Source: CAD feature listing. Evaluate the final solid. Frame: model axes, mm. A direction names the side the tool comes from. Round coordinates to 2 decimals unless told otherwise and drop trailing zeros. Order: outer loops, then holes, each group sorted by start corner. A loop starts at its lowest first (then second) coordinate and runs counter-clockwise, first axis right, second up. Notation, with made-up numbers: (52.5, -1) - (65.5, -1) arc R21 ccw to (65.5, 37) - close; hole circle Ø11 at (78.25, -1). An arc over 180 degrees is marked (long way). Put each result on its own line as item: value. Start each with the question number.
1) Access query for faces 4 (the face through (-91, 10, 7)), 5 (the face through (-100, 5, -2.95)), 6 (the face through (-19.27, 111.66, -4.77)), 7 (the face through (-6, 113, -5)), 8 (the face through (-79.817, 26.321, -17.469)). Directions: +Z, -Z, +X, -X, +Y, -Y. A direction counts if a zero-diameter tool reaches every point of the face in a straight line with its end or side. Return the directions, or none.
2) Contact query for flat-ended pins moving along their axis: P1, Ø1.5, axis at x = -100.5, z = 8, coming from the -Y side; P2, Ø8, axis at y = 94.5, z = -17, coming from the +X side; P3, Ø5, axis at y = 87.25, z = -5, coming from the -X side; P4, Ø10, axis at y = 35.5, z = 1.5, coming from the -X side. Output: stop coordinate, or through.
3) Line query: probe 1 along Y at (x, z) = (-4, 5); probe 2 along X at (y, z) = (9, 4.5); probe 3 along X at (y, z) = (62, 0). Output: solid intervals per line, ascending. Write a range as [from, to].
4) Section B-B on y = 98.5. Output: boundary loops of the cut face in (x, z), then the cut area to 3 significant figures.
5) Section D-D on x = -8.5. Output: boundary loops of the cut face in (y, z).
6) Section C-C on z = -33. Output: boundary loops of the cut face in (x, y), then the cut area to 3 significant figures.
7) Section A-A on z = -8.5. Output: boundary loops of the cut face in (x, y).
8) Mould query, pull axis Z, two halves, no side actions, for faces 1 (the face through (-20.288, 115.135, -4.709)), 2 (the face through (-91, 10, -6)), 3 (the face through (-100, 5, 2.95)). Classes: +Z half, -Z half, draft (parallel to the pull), parting line (faces both ways), or undercut.
```python
from build123d import *

# Parameters (mm, degrees)
BOSS_EXTRUDE1_DEPTH        = 10
SKETCH2_W                  = 5.05
SKETCH2_H                  = 7.05
CUT_EXTRUDE6_DEPTH         = 10
CUT_EXTRUDE7_DEPTH         = 5
CHAMFER2_SIZE              = 5.196152423
CHAMFER2_SIZE_2            = 9
CHAMFER2_OF_MIRROR4_SIZE   = 5.196152423
CHAMFER2_OF_MIRROR4_SIZE_2 = 9
SKETCH5_R                  = 2
CUT_EXTRUDE5_DEPTH         = 6
CUT_EXTRUDE8_START         = -120
CUT_EXTRUDE8_DEPTH         = 24.374622763
SKETCH8_R                  = 144.95
CUT_EXTRUDE9_DEPTH         = 12
BOSS_EXTRUDE2_DEPTH        = 20
SKETCH12_R                 = 2
CUT_EXTRUDE10_DEPTH        = 6
BOSS_EXTRUDE3_START        = -21
SKETCH13_W                 = 31.497171345
SKETCH13_H                 = 26
BOSS_EXTRUDE3_DEPTH        = 4
CHAMFER3_SIZE              = 15


# Read off the part's stored shape, not the designer's step: Cut-Extrude8
with BuildPart() as part:
    # Sketch1 → Boss-Extrude1 (new, symmetric)
    with BuildSketch(Plane.XY):
        Polygon((0, 120), (0, 80), (-10, 80), (-87.75, 12), (-87.75, 0), (-102.75, 0), (-102.75, 24), (-20, 120), align=None)
    extrude(amount=BOSS_EXTRUDE1_DEPTH, both=True)

    # Sketch2 → Cut-Extrude6 (cut)
    with BuildSketch(Plane.XZ):
        with Locations((-100.225, 6.475)):
            Rectangle(SKETCH2_W, SKETCH2_H)
        with Locations((-90.275, 6.475)):
            Rectangle(SKETCH2_W, SKETCH2_H)
        with Locations((-90.275, -6.475)):
            Rectangle(SKETCH2_W, SKETCH2_H)
        with Locations((-100.225, -6.475)):
            Rectangle(SKETCH2_W, SKETCH2_H)
    extrude(amount=-CUT_EXTRUDE6_DEPTH, mode=Mode.SUBTRACT)

    # Sketch6 → Cut-Extrude7 (cut)
    with BuildSketch(Plane.XY.offset(10)):
        Polygon((-98.494242528, 28.937192959), (-85.75, 13.749196141), (-13, 77.376205788), (-25.986145629, 113.055347669), align=None)
    cut_extrude7 = extrude(amount=-CUT_EXTRUDE7_DEPTH, mode=Mode.SUBTRACT)

    # Chamfer2
    # the kernel refuses this chamfer: 9, 5.196152423 mm, written as the material it adds along each edge
    with BuildSketch(Plane(origin=(-5.036481035, 55.496617251, 5), x_dir=(0.05440243528858507, 0.019800867116638043, 0.9983227437537925), z_dir=(-0.342020143325666, 0.9396926207859094, 0))) as chamfer2_piece_1_section:
        Polygon((CHAMFER2_SIZE * 0.998322743697, -CHAMFER2_SIZE * 0.0578938623994), (-CHAMFER2_SIZE_2 * 0.0578938624027, -CHAMFER2_SIZE_2 * 0.998322743754), (0, 0), align=None)
    chamfer2_piece_1 = extrude(amount=84.536493315, mode=Mode.PRIVATE)
    chamfer2_piece_1 = split(chamfer2_piece_1, bisect_by=Plane(origin=(-21.83844233, 92.842389445, 10), z_dir=(0, 0, -1)), keep=Keep.TOP, mode=Mode.PRIVATE)
    chamfer2_piece_1 = split(chamfer2_piece_1, bisect_by=Plane(origin=(-34.214088998, 103.509939047, 6.650101228), z_dir=(0.7574435982041207, -0.6529006015769894, 0)), keep=Keep.TOP, mode=Mode.PRIVATE)
    chamfer2_piece_1 = split(chamfer2_piece_1, bisect_by=Plane(origin=(-10.343648825, 79.699445401, 6.650101228), z_dir=(-0.6583332390976693, 0.7527266079388791, 0)), keep=Keep.TOP, mode=Mode.PRIVATE)
    add(chamfer2_piece_1)
    with BuildSketch(Plane(origin=(-113.460762542, 46.773596955, 5), x_dir=(-0.04434927158426045, -0.03721345742933334, 0.9983227437537927), z_dir=(0.642787609686533, -0.7660444431189835, 0))) as chamfer2_piece_2_section:
        Polygon((CHAMFER2_SIZE * 0.998322743697, -CHAMFER2_SIZE * 0.0578938623994), (-CHAMFER2_SIZE_2 * 0.0578938624027, -CHAMFER2_SIZE_2 * 0.998322743754), (0, 0), align=None)
    chamfer2_piece_2 = extrude(amount=66.394065339, mode=Mode.PRIVATE)
    chamfer2_piece_2 = split(chamfer2_piece_2, bisect_by=Plane(origin=(-97.520772346, 30.066536009, 6.631431033), z_dir=(0.7574435982041207, -0.6529006015769894, 0)), keep=Keep.TOP, mode=Mode.PRIVATE)
    chamfer2_piece_2 = split(chamfer2_piece_2, bisect_by=Plane(origin=(-83.277010041, 15.912068389, 6.631431033), z_dir=(-0.6583332390976693, 0.7527266079388791, 0)), keep=Keep.TOP, mode=Mode.PRIVATE)
    chamfer2_piece_2 = split(chamfer2_piece_2, bisect_by=Plane(origin=(-89.945880011, 23.537136627, 10), z_dir=(0, 0, -1)), keep=Keep.TOP, mode=Mode.PRIVATE)
    add(chamfer2_piece_2)

    # Mirror4: Cut-Extrude7 across plane
    add(cut_extrude7.mirror(Plane.XY), mode=Mode.SUBTRACT)

    # Chamfer2 of Mirror4
    # the kernel refuses this chamfer: 9, 5.196152423 mm, written as the material it adds along each edge
    with BuildSketch(Plane(origin=(-5.036481035, 55.496617251, -5), x_dir=(0.05440243528858507, 0.019800867116638043, -0.9983227437537925), z_dir=(-0.342020143325666, 0.9396926207859094, 0))) as chamfer2_of_mirror4_piece_1_section:
        Polygon((CHAMFER2_OF_MIRROR4_SIZE * 0.998322743697, CHAMFER2_OF_MIRROR4_SIZE * 0.0578938623994), (-CHAMFER2_OF_MIRROR4_SIZE_2 * 0.0578938624027, CHAMFER2_OF_MIRROR4_SIZE_2 * 0.998322743754), (0, 0), align=None)
    chamfer2_of_mirror4_piece_1 = extrude(amount=84.536493315, mode=Mode.PRIVATE)
    chamfer2_of_mirror4_piece_1 = split(chamfer2_of_mirror4_piece_1, bisect_by=Plane(origin=(-34.214088998, 103.509939047, -6.650101228), z_dir=(0.7574435982040639, -0.6529006015770552, 0)), keep=Keep.TOP, mode=Mode.PRIVATE)
    chamfer2_of_mirror4_piece_1 = split(chamfer2_of_mirror4_piece_1, bisect_by=Plane(origin=(-10.343648825, 79.699445401, -6.650101228), z_dir=(-0.6583332390977968, 0.7527266079387677, 0)), keep=Keep.TOP, mode=Mode.PRIVATE)
    chamfer2_of_mirror4_piece_1 = split(chamfer2_of_mirror4_piece_1, bisect_by=Plane(origin=(-21.83844233, 92.842389445, -10), z_dir=(0, 0, 1)), keep=Keep.TOP, mode=Mode.PRIVATE)
    add(chamfer2_of_mirror4_piece_1)
    with BuildSketch(Plane(origin=(-113.460762542, 46.773596955, -5), x_dir=(0.7659013618145366, 0.6426675502167433, 0.019326765612700778), z_dir=(0.642787609686533, -0.7660444431189835, 0))) as chamfer2_of_mirror4_piece_2_section:
        Polygon((CHAMFER2_OF_MIRROR4_SIZE_2 * 0.999813220622, -CHAMFER2_OF_MIRROR4_SIZE_2 * 0.0193267656127), (-CHAMFER2_OF_MIRROR4_SIZE * 0.0193267656116, -CHAMFER2_OF_MIRROR4_SIZE * 0.999813220566), (0, 0), align=None)
    chamfer2_of_mirror4_piece_2 = extrude(amount=66.394065339, mode=Mode.PRIVATE)
    chamfer2_of_mirror4_piece_2 = split(chamfer2_of_mirror4_piece_2, bisect_by=Plane(origin=(-97.520772346, 30.066536009, -6.631431033), z_dir=(0.7574435982040639, -0.6529006015770552, 0)), keep=Keep.TOP, mode=Mode.PRIVATE)
    chamfer2_of_mirror4_piece_2 = split(chamfer2_of_mirror4_piece_2, bisect_by=Plane(origin=(-83.277010041, 15.912068389, -6.631431033), z_dir=(-0.6583332390977968, 0.7527266079387677, 0)), keep=Keep.TOP, mode=Mode.PRIVATE)
    chamfer2_of_mirror4_piece_2 = split(chamfer2_of_mirror4_piece_2, bisect_by=Plane(origin=(-89.945880011, 23.537136627, -10), z_dir=(0, 0, 1)), keep=Keep.TOP, mode=Mode.PRIVATE)
    add(chamfer2_of_mirror4_piece_2)

    # Sketch5 → Cut-Extrude5 (cut)
    with BuildSketch(Plane(origin=(0, 0, 0), x_dir=(0, 0, -1), z_dir=(1, 0, 0))):
        with Locations((-5, 112.75)):
            Circle(SKETCH5_R)
        with Locations((-5, 87.25)):
            Circle(SKETCH5_R)
        with Locations(Location((5, 87.25, 0), (0, 0, 180))):
            Circle(SKETCH5_R)
        with Locations(Location((5, 112.75, 0), (0, 0, 180))):
            Circle(SKETCH5_R)
    extrude(amount=-CUT_EXTRUDE5_DEPTH, mode=Mode.SUBTRACT)

    # Cut-Extrude8 outline → Cut-Extrude8 (cut)
    with BuildSketch(Plane(origin=(0, 120, 0), x_dir=(1, 0, 0), z_dir=(0, 1, 0)).offset(CUT_EXTRUDE8_START)):
        with BuildLine():
            Line((-102.75, 7.56e-07), (-102.75, -10))
            Line((-102.75, -10), (-102.427082983, -10))
            ThreePointArc((-102.427082983, -10), (-102.669249724, -5.002605828), (-102.75, 7.56e-07))
        make_face()
        with BuildLine():
            Line((-102.427082983, 10), (-102.75, 10))
            Line((-102.75, 10), (-102.75, 7.56e-07))
            ThreePointArc((-102.75, 7.56e-07), (-102.669249699, 5.002606583), (-102.427082983, 10))
        make_face()
    extrude(amount=CUT_EXTRUDE8_DEPTH, mode=Mode.SUBTRACT)

    # Sketch8 → Cut-Extrude9 (cut)
    with BuildSketch(Plane.XZ):
        with Locations((56.25, 0)):
            Circle(SKETCH8_R)
    extrude(amount=-CUT_EXTRUDE9_DEPTH, mode=Mode.SUBTRACT)

    # Sketch10 → Boss-Extrude2 (add)
    with BuildSketch(Plane(origin=(0, 0, -10), x_dir=(-1, 0, 0), z_dir=(0, 0, -1))):
        Polygon((87.75, 12), (88.771540348, 10.230640215), (90.560927794, 10.230640215), (90.560927794, 12), align=None)
    extrude(amount=-BOSS_EXTRUDE2_DEPTH)

    # Sketch12 → Cut-Extrude10 (cut)
    with BuildSketch(Plane(origin=(-70.818661801, 61.044211083, 0), x_dir=(0, 0, 1), z_dir=(-0.7574435982041208, 0.6529006015769894, 0))):
        with Locations(Location((-4.797171345, 71.964164649, 0), (0, 0, 270))):
            Circle(SKETCH12_R)
        with Locations(Location((4.797171345, 71.964164649, 0), (0, 0, 90))):
            Circle(SKETCH12_R)
        with Locations(Location((4.797171345, -43.035835351, 0), (0, 0, 270))):
            Circle(SKETCH12_R)
        with Locations(Location((-4.797171345, -43.035835351, 0), (0, 0, 90))):
            Circle(SKETCH12_R)
    extrude(amount=-CUT_EXTRUDE10_DEPTH, mode=Mode.SUBTRACT)

    # Sketch13 → Boss-Extrude3 (add)
    with BuildSketch(Plane(origin=(-70.818661801, 61.044211083, 0), x_dir=(0, 0, 1), z_dir=(-0.7574435982041208, 0.6529006015769894, 0)).offset(BOSS_EXTRUDE3_START)):
        with Locations((-20.748585673, -19.175835351)):
            Rectangle(SKETCH13_W, SKETCH13_H)
    extrude(amount=BOSS_EXTRUDE3_DEPTH)

    # Chamfer3
    chamfer3_edges = [part.edges().sort_by_distance(p)[0] for p in [
        (-70.462035068, 35.42028713, -5),
    ]]
    chamfer(chamfer3_edges, length=CHAMFER3_SIZE)


solid = part.part
```
Answer sheet:
1. face 4: +Z, +X, -Y
1. face 5: -Z, -X, -Y
1. face 6: none
1. face 7: +X
1. face 8: -Z
2. P1: y = 10
2. P2: through
2. P3: x = -50.38
2. P4: x = -97.15
3. probe 1: [80, 85.25], [89.25, 110.75], [114.75, 120]
3. probe 2: [-97.7, -92.8]
3. probe 3: [-69.99, -30.58]
4. outline: (-38.53, -5) - (-30.27, -5) - (-21.05, -10) - (0, -10) - (0, 10) - (-21.05, 10) - (-30.27, 5) - (-38.53, 5) - close
4. area: 642 mm^2
5. outline: (80, -10) - (120, -10) - (120, 10) - (80, 10) - close
6. outline: (-78.95, 25.57) - (-75.92, 22.96) - (-58.94, 42.66) - (-61.97, 45.27) - close
6. area: 104 mm^2
7. outline: (-102.52, 10) - (-97.7, 10) - (-97.7, 0) - (-92.8, 0) - (-92.8, 10) - (-88.45, 10) - (-88.45, 10.79) - (-87.75, 12) - (-83.54, 15.68) - (-96.55, 31.19) - (-102.52, 24.27) - close; (-87.66, 33.08) - (-75.92, 22.96) - (-58.94, 42.66) - (-70.68, 52.78) - close; (-28.18, 110.51) - (-15.37, 75.3) - (-10, 80) - (0, 80) - (0, 120) - (-20, 120) - close
8. face 1: undercut
8. face 2: draft
8. face 3: +Z half
